Can you work these out from the model? Positions are in its coordinate system, mm. A direction names the side the tool comes from. Round coordinates to 2 decimals unless told otherwise and drop trailing zeros. Write each loop counter-clockwise with the first axis right and the second up, starting at its lowest first coordinate (ties: lowest second). Pieces come first, ordered by that corner, then holes.
Q1. For faces 4 (the cylindrical face through (-22.57, -0.65, 4.48)), 5 (the cylindrical face through (27, 0, 1)), which set-ups out of +Z, -Z, +X, -X, +Y, -Y let a thin tool reach every point of the face, with its end or its side?
Q2. Please list where these lines run through material, in increasing order: line 1 along Y through (x, z) = (0, 5.35); line 2 along X through (y, z) = (-18.5, 5.3); line 3 along Y through (x, z) = (-23, 4.1).
Q3. I'm going to push flat-ended pins straight in: pin 1 Ø1 at (x, z) = (8, 5) entering from +Y; pin 2 Ø1 at (y, z) = (-9, 4.5) entering from +X; pin 3 Ø1.5 at (y, z) = (-27, 3.5) entering from -X. Where does each tip first touch, or does it pass through?
Q4. If we section it at D-D (y = -8): Please give me the cut outline in (x, z), plus the area to 3 significant figures.
Q5. If we section it at A-A (y = 0): Please give me the cut outline in (x, z), plus the area to 3 significant figures.
Q6. If we section it at C-C (x = -25.5): Please give me the cut outline in (y, z).
Q7. We'd pull the mould along Y, two halves only. Please class faces 1 (the flat face through (-20, 19, 3)), 2 (the flat face through (0, 0, 6)), 3 (the cylindrical face through (18.28, 28.67, 2.96)): +Y half, -Y half, draft (parallel to the pull), parting line (faces both ways), or undercut.
from build123d import *

# Parameters (mm, degrees)
CYLINDER796_R                = 1.5
CYLINDER796_DEPTH            = 20
CYLINDER796_PLACEMENT_ANGLE  = 45
CYLINDER797_R                = 1.5
CYLINDER797_DEPTH            = 20
CYLINDER798_R                = 1.5
CYLINDER798_DEPTH            = 20
CYLINDER798_PLACEMENT_ANGLE  = 135
CYLINDER799_R                = 1.5
CYLINDER799_DEPTH            = 20
CYLINDER800_R                = 1.5
CYLINDER800_DEPTH            = 20
CYLINDER800_PLACEMENT_ANGLE  = 225
CYLINDER801_R                = 1.5
CYLINDER801_DEPTH            = 20
CYLINDER802_R                = 1.5
CYLINDER802_DEPTH            = 20
CYLINDER802_PLACEMENT_ANGLE  = 45
CYLINDER794_R                = 1.5
CYLINDER794_DEPTH            = 20
CYLINDER803_R                = 3
CYLINDER803_DEPTH            = 3
CYLINDER803_PLACEMENT_ANGLE  = 45
CYLINDER1815_R               = 3
CYLINDER1815_DEPTH           = 3
CYLINDER1814_R               = 3
CYLINDER1814_DEPTH           = 3
CYLINDER1814_PLACEMENT_ANGLE = 135
CYLINDER1806_R               = 3
CYLINDER1806_DEPTH           = 3
CYLINDER1810_R               = 3
CYLINDER1810_DEPTH           = 3
CYLINDER1810_PLACEMENT_ANGLE = 225
CYLINDER1807_R               = 3
CYLINDER1807_DEPTH           = 3
CYLINDER1808_R               = 3
CYLINDER1808_DEPTH           = 3
CYLINDER1808_PLACEMENT_ANGLE = 45
CYLINDER795_R                = 3
CYLINDER795_DEPTH            = 3
CYLINDER257_R                = 34
CYLINDER257_DEPTH            = 6


with BuildPart() as obj1:
    # Cylinder796 → Cylinder796 (new body)
    with BuildSketch(Plane.XY):
        Circle(CYLINDER796_R)
    extrude(amount=CYLINDER796_DEPTH)


with BuildPart() as obj1_1:
    # Cylinder796 placement: moved
    add(obj1.part.moved(Location((-18.031223, 18.031223, -4))).rotate(Axis((-18.031223, 18.031223, -4), (0, 0, 1)), CYLINDER796_PLACEMENT_ANGLE))


with BuildPart() as obj2:
    # Cylinder797 → Cylinder797 (new body)
    with BuildSketch(Plane(origin=(-25.5, 0, -4), x_dir=(0, 1, 0), z_dir=(0, 0, 1))):
        Circle(CYLINDER797_R)
    extrude(amount=CYLINDER797_DEPTH)


with BuildPart() as obj3:
    # Cylinder798 → Cylinder798 (new body)
    with BuildSketch(Plane.XY):
        Circle(CYLINDER798_R)
    extrude(amount=CYLINDER798_DEPTH)


with BuildPart() as obj3_1:
    # Cylinder798 placement: moved
    add(obj3.part.moved(Location((-18.031223, -18.031223, -4))).rotate(Axis((-18.031223, -18.031223, -4), (0, 0, 1)), CYLINDER798_PLACEMENT_ANGLE))


with BuildPart() as obj4:
    # Cylinder799 → Cylinder799 (new body)
    with BuildSketch(Plane(origin=(0, -25.5, -4), x_dir=(-1, 0, 0), z_dir=(0, 0, 1))):
        Circle(CYLINDER799_R)
    extrude(amount=CYLINDER799_DEPTH)


with BuildPart() as obj5:
    # Cylinder800 → Cylinder800 (new body)
    with BuildSketch(Plane.XY):
        Circle(CYLINDER800_R)
    extrude(amount=CYLINDER800_DEPTH)


with BuildPart() as obj5_1:
    # Cylinder800 placement: moved
    add(obj5.part.moved(Location((18.031223, -18.031223, -4))).rotate(Axis((18.031223, -18.031223, -4), (0, 0, 1)), CYLINDER800_PLACEMENT_ANGLE))


with BuildPart() as obj6:
    # Cylinder801 → Cylinder801 (new body)
    with BuildSketch(Plane(origin=(25.5, 0, -4), x_dir=(0, -1, 0), z_dir=(0, 0, 1))):
        Circle(CYLINDER801_R)
    extrude(amount=CYLINDER801_DEPTH)


with BuildPart() as obj7:
    # Cylinder802 → Cylinder802 (new body)
    with BuildSketch(Plane.XY):
        Circle(CYLINDER802_R)
    extrude(amount=CYLINDER802_DEPTH)


with BuildPart() as obj7_1:
    # Cylinder802 placement: moved
    add(obj7.part.moved(Location((18.031223, 18.031223, -4))).rotate(Axis((18.031223, 18.031223, -4), (0, 0, -1)), CYLINDER802_PLACEMENT_ANGLE))


with BuildPart() as compound003:
    # Cylinder794 → Cylinder794 (new body)
    with BuildSketch(Plane(origin=(0, 25.5, -4), x_dir=(1, 0, 0), z_dir=(0, 0, 1))):
        Circle(CYLINDER794_R)
    extrude(amount=CYLINDER794_DEPTH)

    # Compound003: union obj1, obj2, obj3, obj4, obj5, obj6, obj7
    add(obj1_1.part)
    add(obj2.part)
    add(obj3_1.part)
    add(obj4.part)
    add(obj5_1.part)
    add(obj6.part)
    add(obj7_1.part)


with BuildPart() as obj8:
    # Cylinder803 → Cylinder803 (new body)
    with BuildSketch(Plane.XY):
        Circle(CYLINDER803_R)
    extrude(amount=CYLINDER803_DEPTH)


with BuildPart() as obj8_1:
    # Cylinder803 placement: moved
    add(obj8.part.moved(Location((-18.031223, 18.031223, 3))).rotate(Axis((-18.031223, 18.031223, 3), (0, 0, 1)), CYLINDER803_PLACEMENT_ANGLE))


with BuildPart() as obj9:
    # Cylinder1815 → Cylinder1815 (new body)
    with BuildSketch(Plane(origin=(-25.5, 0, 3), x_dir=(0, 1, 0), z_dir=(0, 0, 1))):
        Circle(CYLINDER1815_R)
    extrude(amount=CYLINDER1815_DEPTH)


with BuildPart() as obj10:
    # Cylinder1814 → Cylinder1814 (new body)
    with BuildSketch(Plane.XY):
        Circle(CYLINDER1814_R)
    extrude(amount=CYLINDER1814_DEPTH)


with BuildPart() as obj10_1:
    # Cylinder1814 placement: moved
    add(obj10.part.moved(Location((-18.031223, -18.031223, 3))).rotate(Axis((-18.031223, -18.031223, 3), (0, 0, 1)), CYLINDER1814_PLACEMENT_ANGLE))


with BuildPart() as obj11:
    # Cylinder1806 → Cylinder1806 (new body)
    with BuildSketch(Plane(origin=(0, -25.5, 3), x_dir=(-1, 0, 0), z_dir=(0, 0, 1))):
        Circle(CYLINDER1806_R)
    extrude(amount=CYLINDER1806_DEPTH)


with BuildPart() as obj12:
    # Cylinder1810 → Cylinder1810 (new body)
    with BuildSketch(Plane.XY):
        Circle(CYLINDER1810_R)
    extrude(amount=CYLINDER1810_DEPTH)


with BuildPart() as obj12_1:
    # Cylinder1810 placement: moved
    add(obj12.part.moved(Location((18.031223, -18.031223, 3))).rotate(Axis((18.031223, -18.031223, 3), (0, 0, 1)), CYLINDER1810_PLACEMENT_ANGLE))


with BuildPart() as obj13:
    # Cylinder1807 → Cylinder1807 (new body)
    with BuildSketch(Plane(origin=(25.5, 0, 3), x_dir=(0, -1, 0), z_dir=(0, 0, 1))):
        Circle(CYLINDER1807_R)
    extrude(amount=CYLINDER1807_DEPTH)


with BuildPart() as obj14:
    # Cylinder1808 → Cylinder1808 (new body)
    with BuildSketch(Plane.XY):
        Circle(CYLINDER1808_R)
    extrude(amount=CYLINDER1808_DEPTH)


with BuildPart() as obj14_1:
    # Cylinder1808 placement: moved
    add(obj14.part.moved(Location((18.031223, 18.031223, 3))).rotate(Axis((18.031223, 18.031223, 3), (0, 0, -1)), CYLINDER1808_PLACEMENT_ANGLE))


with BuildPart() as compound004:
    # Cylinder795 → Cylinder795 (new body)
    with BuildSketch(Plane(origin=(0, 25.5, 3), x_dir=(1, 0, 0), z_dir=(0, 0, 1))):
        Circle(CYLINDER795_R)
    extrude(amount=CYLINDER795_DEPTH)

    # Compound004: union obj8, obj9, obj10, obj11, obj12, obj13, obj14
    add(obj8_1.part)
    add(obj9.part)
    add(obj10_1.part)
    add(obj11.part)
    add(obj12_1.part)
    add(obj13.part)
    add(obj14_1.part)


with BuildPart() as cut003:
    # Cylinder257 → Cylinder257 (new body)
    with BuildSketch(Plane.XY):
        Circle(CYLINDER257_R)
    extrude(amount=CYLINDER257_DEPTH)

    # Cut002: cut Compound004
    add(compound004.part, mode=Mode.SUBTRACT)

    # Cut003: cut Compound003
    add(compound003.part, mode=Mode.SUBTRACT)


solid = cut003.part
A:
1. face 4: +Z
1. face 5: +Z, -Z
2. line 1: y = -34 to -28.5, -22.5 to 22.5, 28.5 to 34
2. line 2: x = -28.53 to -20.99, -15.07 to 15.07, 20.99 to 28.53
2. line 3: y = -25.04 to -1.66, 1.66 to 25.04
3. pin 1: stops at y = 33.16
3. pin 2: stops at x = 32.92
3. pin 3: stops at x = -21.61
4. outline: (-33.05, 0) - (33.05, 0) - (33.05, 6) - (-33.05, 6) - close
4. area: 397 mm2
5. outline: (-34, 0) - (-27, 0) - (-27, 3) - (-28.5, 3) - (-28.5, 6) - (-34, 6) - close; (-24, 0) - (24, 0) - (24, 3) - (22.5, 3) - (22.5, 6) - (-22.5, 6) - (-22.5, 3) - (-24, 3) - close; (27, 0) - (34, 0) - (34, 6) - (28.5, 6) - (28.5, 3) - (27, 3) - close
5. area: 354 mm2
6. outline: (-22.49, 0) - (-1.5, 0) - (-1.5, 3) - (-3, 3) - (-3, 6) - (-22.49, 6) - close; (1.5, 0) - (22.49, 0) - (22.49, 6) - (3, 6) - (3, 3) - (1.5, 3) - close
7. face 1: undercut
7. face 2: draft
7. face 3: parting line
